Build history of the part. All positions in model axes, mm. Give positions to 0.01 mm unless a question says otherwise; leave off trailing zeros. Order: outer loops, then holes, each group sorted by start corner. A loop starts at its lowest first (then second) coordinate and runs counter-clockwise, first axis right, second up. Notation, with made-up numbers: (54.5, 6) - (73.5, 6) arc R25 ccw to (73.5, 35) - close; hole circle Ø2 at (31.5, 83). An arc over 180 degrees is marked (long way). Use a Markdown table: item, result.
from build123d import *

# Parameters (mm, degrees)
BASE_FLANGE1_DEPTH = 1
FILLET1_R          = 3
SKETCH2_R          = 3
CUT_EXTRUDE1_DEPTH = 10


# Sheet-metal steps are written as plain solids
with BuildPart() as part:
    # Sketch1 → Base-Flange1 (new body)
    with BuildSketch(Plane.XY):
        Polygon((0, 0), (0, 237.736706628), (412, 475.605017534), (412, 580.417185402), (-91, 290.01), (-91, 0), align=None)
    extrude(amount=-BASE_FLANGE1_DEPTH)

    # Fillet1
    fillet1_edges = [part.edges().sort_by_distance(p)[0] for p in [
        (-91, 0, -0.5),
        (-91, 290.01, -0.5),
        (412, 580.417185402, -0.5),
        (412, 475.605017534, -0.5),
        (0, 237.736706628, -0.5),
        (0, 0, -0.5),
    ]]
    fillet(fillet1_edges, radius=FILLET1_R)

    # Sketch2 → Cut-Extrude1 (cut)
    with BuildSketch(Plane(origin=(0, 0, -1), x_dir=(-1, 0, 0), z_dir=(0, 0, -1))):
        with Locations((-382, 556.168474096)):
            Circle(SKETCH2_R)
        with Locations((-240.404846481, 474.418474096)):
            Circle(SKETCH2_R)
        with Locations((-98.809692962, 392.668474096)):
            Circle(SKETCH2_R)
        with Locations((42.785460556, 310.918474096)):
            Circle(SKETCH2_R)
        with Locations((-382, 465.212712688)):
            Circle(SKETCH2_R)
        with Locations((-267.6846467, 399.212712688)):
            Circle(SKETCH2_R)
        with Locations((-153.369293401, 333.212712688)):
            Circle(SKETCH2_R)
        with Locations((-39.053940101, 267.212712688)):
            Circle(SKETCH2_R)
        with Locations((85, 30)):
            Circle(SKETCH2_R)
        with Locations((6, 40)):
            Circle(SKETCH2_R)
        with Locations((85, 140)):
            Circle(SKETCH2_R)
        with Locations((85, 250)):
            Circle(SKETCH2_R)
        with Locations((6, 205)):
            Circle(SKETCH2_R)
    extrude(amount=-CUT_EXTRUDE1_DEPTH, mode=Mode.SUBTRACT)


solid = part.part
1) Wall check: line 1 (Y direction, x = -6, z = -0.3); line 2 (X direction, y = 140, z = -0.45); line 3 (Y direction, x = 382, z = -0.4). Give the ranges that are in metal, low to high. Write a range as from..to.
Computed:
| item | result |
|---|---|
| line 1 | y = 0..37, 43..202, 208..339.08 |
| line 2 | x = -91..-88, -82..0 |
| line 3 | y = 458.28..462.21, 468.21..553.17, 559.17..563.1 |
2) Slice it at B-B (x = -15.5). Write the cut outline in (y, z).
Computed:
| item | result |
|---|---|
| outline | (0, -1) - (333.6, -1) - (333.6, 0) - (0, 0) - close |
3) Slice it at A-A (z = -0.6). State how many separate pieces and enclosed holes the cut face has, and give its area (3 significant figures).
Computed:
| item | result |
|---|---|
| separate pieces | 1 |
| enclosed holes | 13 |
| area | 71,600 mm² |
4) Slice it at C-C (y = 543). Write the cut outline in (x, z), and give its area (3 significant figures).
Computed:
| item | result |
|---|---|
| outline | (347.19, -1) - (412, -1) - (412, 0) - (347.19, 0) - close |
| area | 64.8 mm² |
5) Pin check, flat tips, straight feed: P1, Ø9.5, axis at x = 153.37, y = 333.21, coming from the -Z side; P2, Ø0.5, axis at y = 168, z = -0.5, coming from the +X side. Stop position of each tip, or through.
Computed:
| item | result |
|---|---|
| P1 | stops at z = -1 |
| P2 | stops at x = 0 |
